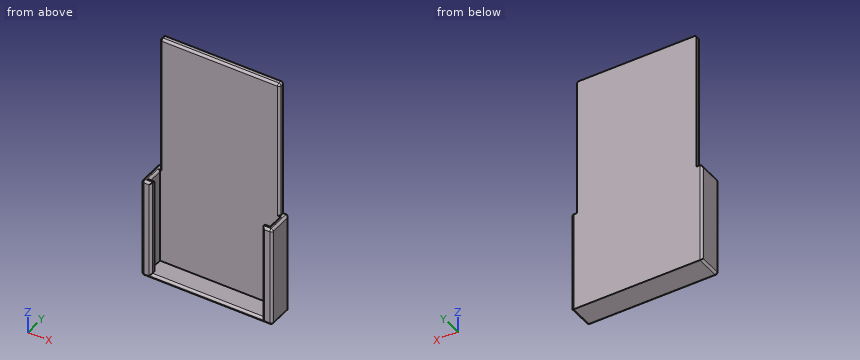
```python
from build123d import *

# Parameters (mm, degrees)
F0_W     = 61
F0_H     = 12
F0_W_2   = 56
F0_H_2   = 7
F1_DEPTH = 45
F2_W     = 52
F2_H     = 45
F3_DEPTH = 3
F4_W     = 61
F4_H     = 12
F5_DEPTH = 2
F6_W     = 56
F6_H     = 2.5
F7_DEPTH = 65
F8_R     = 0.99999
F9_R     = 0.99999


# Not quite as in the source:
# - a fillet or chamfer is up to 0.001 mm smaller than in the source, because OpenCascade refuses the exact size


with BuildPart() as f1:
    # F0 (on Top) → F1 (new body)
    with BuildSketch(Plane.XY):
        Rectangle(F0_W, F0_H)
        Rectangle(F0_W_2, F0_H_2, mode=Mode.SUBTRACT)
    extrude(amount=F1_DEPTH)

    # F2 (on face) → F3 (cut)
    with BuildSketch(Plane.XZ.offset(6)):
        with Locations((0, 22.5)):
            Rectangle(F2_W, F2_H)
    extrude(amount=-F3_DEPTH, mode=Mode.SUBTRACT)

    # F4 (on face) → F5 (join)
    with BuildSketch(Plane(origin=(0, 0, 0), x_dir=(1, 0, 0), z_dir=(0, 0, -1))):
        Rectangle(F4_W, F4_H)
    extrude(amount=F5_DEPTH)

    # F6 (on face) → F7 (join)
    with BuildSketch(Plane.XY.offset(45)):
        with Locations((0, 4.75)):
            Rectangle(F6_W, F6_H)
    extrude(amount=F7_DEPTH)

    # F8 (radius 1 in the source; OpenCascade refuses exactly that, so slightly less here)
    f8_edges = [f1.edges().sort_by_distance(p)[0] for p in [
        (-26, -6, 22.5),
        (0, -6, 0),
        (26, -6, 22.5),
        (28.25, -6, 45),
        (30.5, -6, 21.5),
        (0, -6, -2),
        (-30.5, -6, 21.5),
        (-28.25, -6, 45),
        (-28, 0, 45),
        (28, 0, 45),
        (27, -3.5, 45),
        (-27, -3.5, 45),
        (-30.5, 0, 45),
        (30.5, 0, 45),
        (30.5, 6, 21.5),
        (30.5, 0, -2),
        (-30.5, 6, 21.5),
        (-30.5, 0, -2),
        (0, 3.5, 110),
    ]]
    fillet(f8_edges, radius=F8_R)

    # F9 (radius 1 in the source; OpenCascade refuses exactly that, so slightly less here)
    f9_edges = [f1.edges().sort_by_distance(p)[0] for p in [
        (-28, 3.5, 77.000005),
        (28, 3.5, 77.000005),
    ]]
    fillet(f9_edges, radius=F9_R)


solid = f1.part
```
Geometry: final body of the model. Coordinates: model frame, mm. Give positions to 0.01 mm unless a question says otherwise; leave off trailing zeros. Write each loop counter-clockwise with the first axis right and the second up, starting at its lowest first coordinate (ties: lowest second). Pieces come first, ordered by that corner, then holes.
1. Pin query (flat end, axial travel): P1, Ø1.8, axis at x = 28, y = 0, coming from the +Z side (3 decimals); P2, Ø1.2, axis at y = 5.5, z = 63, coming from the -X side; P3, Ø4, axis at x = 9, y = -0.5, coming from the +Z side. Return the tip coordinate at first contact, or that it passes through.
2. Section query D-D, the plane z = 96. Return loops of the section in (x, y), then the cut area to 3 significant figures.
3. Section query C-C, the plane z = 30. Return loops of the section in (x, y), then the cut area to 3 significant figures.
4. Section query B-B, the plane y = 1. Return loops of the section in (x, z), then the cut area to 3 significant figures.
5. Line query: probe 1 along X at (y, z) = (2.75, 15); probe 2 along Z at (x, y) = (-14, -0.5); probe 3 along Y at (x, z) = (-6, 97.5). Output: solid intervals per line, ascending.
Computed:
1. P1: stops at z = 44.995
1. P2: stops at x = -28
1. P3: stops at z = 0
2. outline: (-28, 4.5) arc R1 ccw to (-27, 3.5) - (27, 3.5) arc R1 ccw to (28, 4.5) - (28, 6) - (-28, 6) - close
2. area: 140 mm2
3. outline: (-30.5, -5) arc R1 ccw to (-29.5, -6) - (-27, -6) arc R1 ccw to (-26, -5) - (-26, -3.5) - (-28, -3.5) - (-28, 3.5) - (28, 3.5) - (28, -3.5) - (26, -3.5) - (26, -5) arc R1 ccw to (27, -6) - (29.5, -6) arc R1 ccw to (30.5, -5) - (30.5, 5) arc R1 ccw to (29.5, 6) - (-29.5, 6) arc R1 ccw to (-30.5, 5) - close
3. area: 209 mm2
4. outline: (-30.5, -1) arc R1 ccw to (-29.5, -2) - (29.5, -2) arc R1 ccw to (30.5, -1) - (30.5, 44) arc R1 ccw to (29.5, 45) - (29, 45) arc R1 ccw to (28, 44) - (28, 0) - (-28, 0) - (-28, 44) arc R1 ccw to (-29, 45) - (-29.5, 45) arc R1 ccw to (-30.5, 44) - close
4. area: 346 mm2
5. probe 1: x = -30.5 to -28, 28 to 30.5
5. probe 2: z = -2 to 0
5. probe 3: y = 3.5 to 6
